CAD build for the part. Positions are in the model's coordinates, mm. Face numbers are marked on the shaded views. A direction names the side the tool comes from. Round coordinates to 2 decimals unless told otherwise and drop trailing zeros. Write each loop counter-clockwise with the first axis right and the second up, starting at its lowest first coordinate (ties: lowest second). Pieces come first, ordered by that corner, then holes. Notation, with made-up numbers: M 82.25,-7.75 L 102.25,-7.75 A36 ccw 102.25,26.25 Z; hole C 70.5,44 d7. An arc over 180 degrees is marked long. Write each question's results on one line, items separated by ' | '. Start each with the question number.
```python
from build123d import *

# Parameters (mm, degrees)
SKETCH1_R               = 31.34
BOSS_EXTRUDE1_DEPTH     = 200
SKETCH2_R               = 37.5
BOSS_EXTRUDE2_DEPTH     = 265
CUT_EXTRUDE1_DEPTH      = 469.014422855
CUT_EXTRUDE1_DEPTH_BACK = 469.014422855
SKETCH3_R               = 11


with BuildPart() as part:
    # Sketch1 → Boss-Extrude1 (new body)
    with BuildSketch(Plane.XY):
        Circle(SKETCH1_R)
    extrude(amount=BOSS_EXTRUDE1_DEPTH)

    # Sketch2 → Boss-Extrude2 (add)
    with BuildSketch(Plane.XY.offset(200)):
        Circle(SKETCH2_R)
    extrude(amount=BOSS_EXTRUDE2_DEPTH)

    # Sketch3 → Cut-Extrude1 (cut, two sides: drawn at the far end of the back side and taken through both)
    with BuildSketch(Plane(origin=(0, 0, 0), x_dir=(1, 0, 0), z_dir=(0, 1, 0)).offset(-CUT_EXTRUDE1_DEPTH_BACK)):
        with Locations(Location((0, -150, 0), (0, 0, 270))):
            Circle(SKETCH3_R)
        with Locations(Location((0, -50, 0), (0, 0, 270))):
            Circle(SKETCH3_R)
    extrude(amount=CUT_EXTRUDE1_DEPTH + CUT_EXTRUDE1_DEPTH_BACK, mode=Mode.SUBTRACT)


solid = part.part
```
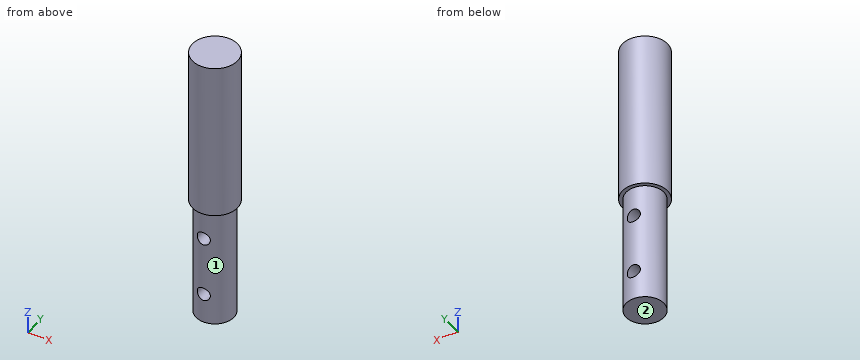
1) Wall check: line 1 along Z through (x, y) = (0, -8); line 2 along X through (y, z) = (1, 150); line 3 along Z through (x, y) = (6.5, 11.5). Give the ranges that are in metal, low to high. Write a range as from..to.
2) 3-axis set-ups, long thin cutter, end or side, ignore diameter. For the marked faces 1 and 2: which of +Z, -Z, +X, -X, +Y, -Y reach the whole face in a straight line?
3) Saw through at D-D, the plane z = 150. Write the cut outline in (x, y), plus the area to 3 significant figures.
4) Saw through at A-A, the plane x = 0. Write the cut outline in (y, z).
5) Saw through at C-C, the plane z = 31.5. Write the cut outline in (x, y).
6) Saw through at B-B, the plane y = 0. Write the cut outline in (x, z).
7) Drop flat-ended pins along their axis: pin 1 Ø1.5 at (y, z) = (-2.5, 275) entering from +X; pin 2 Ø1.5 at (x, y) = (24, -21.5) entering from -Z; pin 3 Ø3 at (y, z) = (14, 395) entering from +X; pin 4 Ø17.5 at (x, z) = (0, 50) entering from -Y. Give the stop position or say it passes through.
Filled sheet:
1) line 1: z = 0..39, 61..139, 161..465 | line 2: x = -31.32..-11, 11..31.32 | line 3: z = 0..41.13, 58.87..141.13, 158.87..465
2) face 1: -Z | face 2: -Z, +X, -X, +Y, -Y
3) outline: M -11,-29.35 L -11,29.35 A31.34 ccw Z; M 11,-29.35 A31.34 ccw 11,29.35 Z | area: 1,740 mm^2
4) outline: M -37.5,200 L -31.34,200 L -31.34,161 L 31.34,161 L 31.34,200 L 37.5,200 L 37.5,465 L -37.5,465 Z; M -31.34,0 L 31.34,0 L 31.34,39 L -31.34,39 Z; M -31.34,61 L 31.34,61 L 31.34,139 L -31.34,139 Z
5) outline: C 0,0 d62.68
6) outline: M -37.5,200 L -31.34,200 L -31.34,0 L 31.34,0 L 31.34,200 L 37.5,200 L 37.5,465 L -37.5,465 Z; hole C 0,50 d22; hole C 0,150 d22
7) pin 1: stops at x = 37.46 | pin 2: stops at z = 200 | pin 3: stops at x = 35.36 | pin 4: passes through
